from build123d import *

# Parameters (mm, degrees)
SKETCH1_W            = 812.8
SKETCH1_H            = 711.2
BOSS_EXTRUDE1_DEPTH  = 152.4
SKETCH2_W            = 609.6
SKETCH2_H            = 508
CUT_EXTRUDE1_DEPTH   = 152.4
SKETCH4_R            = 31.75
BOSS_EXTRUDE3_DEPTH  = 508
BOSS_EXTRUDE4_DEPTH  = 508
SKETCH7_R            = 31.75
BOSS_EXTRUDE5_DEPTH  = 508
BOSS_EXTRUDE6_DEPTH  = 508
BOSS_EXTRUDE7_DEPTH  = 508
SKETCH11_W           = 50.8
SKETCH11_H           = 508
BOSS_EXTRUDE8_DEPTH  = 76.2
CUT_EXTRUDE2_DEPTH   = 508
SKETCH14_W           = 609.6
SKETCH14_H           = 25.4
BOSS_EXTRUDE10_DEPTH = 50.8
SKETCH15_R           = 31.75
BOSS_EXTRUDE11_DEPTH = 508


with BuildPart() as part:
    # Sketch1 → Boss-Extrude1 (new body)
    with BuildSketch(Plane(origin=(0, 0, 0), x_dir=(1, 0, 0), z_dir=(0, 1, 0))):
        with Locations((406.4, -355.6)):
            Rectangle(SKETCH1_W, SKETCH1_H)
    extrude(amount=BOSS_EXTRUDE1_DEPTH)

    # Sketch2 → Cut-Extrude1 (cut)
    with BuildSketch(Plane(origin=(0, 152.4, 0), x_dir=(1, 0, 0), z_dir=(0, 1, 0))):
        with Locations((406.4, -355.6)):
            Rectangle(SKETCH2_W, SKETCH2_H)
    extrude(amount=-CUT_EXTRUDE1_DEPTH, mode=Mode.SUBTRACT)

    # Sketch4 → Boss-Extrude3 (add)
    with BuildSketch(Plane.XY.offset(101.6)):
        with Locations(Location((152.4, 25.4, 0), (0, 0, 233.130102354))):
            Circle(SKETCH4_R)
    extrude(amount=BOSS_EXTRUDE3_DEPTH)

    # Sketch6 → Boss-Extrude4 (add)
    with BuildSketch(Plane.XY.offset(101.6)):
        with BuildLine():
            Line((373.396614636, 28.575), (482.6, 152.4))
            Line((482.6, 152.4), (482.6, 0))
            Line((482.6, 0), (386.295833398, 0))
            ThreePointArc((386.295833398, 0), (382.921614636, 15.675781238), (373.396614636, 28.575))
        make_face()
    extrude(amount=BOSS_EXTRUDE4_DEPTH)

    # Sketch7 → Boss-Extrude5 (add)
    with BuildSketch(Plane.XY.offset(101.6)):
        with Locations(Location((348.195833398, 0, 0), (0, 0, 180))):
            Circle(SKETCH7_R)
    extrude(amount=BOSS_EXTRUDE5_DEPTH)

    # Sketch8 → Boss-Extrude6 (add)
    with BuildSketch(Plane.XY.offset(101.6)):
        Polygon((373.396614636, 28.575), (363.871614636, 36.975260413), (473.075, 160.800260413), (482.6, 152.4), align=None)
    extrude(amount=BOSS_EXTRUDE6_DEPTH)

    # Sketch9 → Boss-Extrude7 (add)
    with BuildSketch(Plane.XY.offset(609.6)):
        Polygon((482.6, 152.4), (641.222949159, 635), (631.697949159, 643.400260413), (473.075, 160.800260413), align=None)
    extrude(amount=-BOSS_EXTRUDE7_DEPTH)

    # Sketch11 → Boss-Extrude8 (add)
    with BuildSketch(Plane(origin=(379.25081554, -124.653714944, 0), x_dir=(0, 0, 1), z_dir=(-0.95, 0.3122498999199199, 0))):
        with Locations((584.2, 554.477868797)):
            Rectangle(SKETCH11_W, SKETCH11_H)
        with Locations((127, 554.477868797)):
            Rectangle(SKETCH11_W, SKETCH11_H)
    extrude(amount=BOSS_EXTRUDE8_DEPTH)

    # Sketch12 → Cut-Extrude2 (cut)
    with BuildSketch(Plane(origin=(0, 0, 101.6), x_dir=(-1, 0, 0), z_dir=(0, 0, -1))):
        Polygon((-579.47237543, 647.197555329), (-429.198002543, 189.997555329), (-453.328002543, 182.066407871), (-603.60237543, 639.266407871), align=None)
    extrude(amount=-CUT_EXTRUDE2_DEPTH, mode=Mode.SUBTRACT)

    # Sketch14 → Boss-Extrude10 (add)
    with BuildSketch(Plane(origin=(0, 152.4, 0), x_dir=(1, 0, 0), z_dir=(0, 1, 0))):
        with Locations((406.4, -88.9)):
            Rectangle(SKETCH14_W, SKETCH14_H)
        with Locations((406.4, -622.3)):
            Rectangle(SKETCH14_W, SKETCH14_H)
    extrude(amount=BOSS_EXTRUDE10_DEPTH)

    # Sketch15 → Boss-Extrude11 (add)
    with BuildSketch(Plane(origin=(0, 0, 609.6), x_dir=(-1, 0, 0), z_dir=(0, 0, -1))):
        with Locations(Location((-342.9, 127, 0), (0, 0, 180))):
            Circle(SKETCH15_R)
    extrude(amount=BOSS_EXTRUDE11_DEPTH)


solid = part.part
Source: CAD feature listing. Evaluate the final solid. Frame: model axes, mm. A direction names the side the tool comes from. Give positions to 0.01 mm unless a question says otherwise; leave off trailing zeros. Loops run counter-clockwise (first coordinate to the right, second up) from the corner with the lowest first, then second, coordinate; pieces in that order, holes last. Notation, with made-up numbers: (75.25, 57.25) -> (87.25, 57.25) arc R25 ccw to (87.25, 71.25) -> close; hole circle Ø4 at (8, -18). An arc over 180 degrees is marked (long way). Use a Markdown table: item, result. Add a question column.
1) First-contact query: pin 1 (3 mm diameter, centred on y = 247, z = 578.5, fed in from -X); pin 2 (2 mm diameter, centred on y = 262.5, z = 561, fed in from +X); pin 3 (1 mm diameter, centred on y = 558.5, z = 579, fed in from -X). Flat tips, straight axial feed; report the tip coordinate or a pass-through.
2) Line query: line 1 along X through (y, z) = (80, 330); line 2 along X through (y, z) = (134, 360); line 3 along Y through (x, z) = (715.5, 325.5). Output: solid intervals per line, ascending. Write a range as [from, to].
3) Section query D-D, the plane y = 127. Return the cut outline in (x, z).
4) Reachability of faces 5 (the face through (711.2, 77, 359)), 6 (the face through (541, 419, 101.6)), 7 (the face through (445, 195, 101.6)), 8 (the face through (101.6, 177, 89)), 9 (the face through (711.2, 177, 622)) from +Z, -Z, +X, -X, +Y, -Y: full face, straight path, thin tool, end or side. Return the list, or none.
5) Pull-direction query (X, two-part tool) for faces 1 (the face through (243, 103, 609.6)), 2 (the face through (505.387, 421.798, 126.644)), 3 (the face through (0, 75, 361)), 4 (the face through (401, 75, 0)); classes: +X half, -X half, draft (parallel to the pull), parting line (faces both ways), or undercut.
6) Section query C-C, the plane y = 399.5. Return the cut outline in (x, z).
7) Section query A-A, the plane x = 689. Return the cut outline in (y, z), then the cut area to 3 significant figures.
8) Section query B-B, the plane z = 331.5. Return the cut outline in (x, y) (3 decimals).
Numbers:
| question | item | result |
|---|---|---|
| 1 | pin 1 | stops at x = 420.7 |
| 1 | pin 2 | stops at x = 519.12 |
| 1 | pin 3 | stops at x = 523.42 |
| 2 | line 1 | x = [0, 101.6], [401.82, 482.6], [711.2, 812.8] |
| 2 | line 2 | x = [0, 101.6], [311.93, 373.87], [449.44, 482.6], [711.2, 812.8] |
| 2 | line 3 | y = [0, 152.4] |
| 3 | outline | (0, 0) -> (812.8, 0) -> (812.8, 711.2) -> (0, 711.2) -> close; hole (101.6, 101.6) -> (311.15, 101.6) -> (311.15, 609.6) -> (101.6, 609.6) -> close; hole (374.65, 101.6) -> (443.27, 101.6) -> (443.27, 609.6) -> (374.65, 609.6) -> close; hole (482.6, 101.6) -> (711.2, 101.6) -> (711.2, 609.6) -> (482.6, 609.6) -> close |
| 4 | face 5 | +Y, -Y |
| 4 | face 6 | -Z, +X, -X, +Y |
| 4 | face 7 | none |
| 4 | face 8 | +Z, -Z, -X, +Y |
| 4 | face 9 | +Z, -Z, +X, +Y |
| 5 | face 1 | undercut |
| 5 | face 2 | undercut |
| 5 | face 3 | -X half |
| 5 | face 4 | draft |
| 6 | outline | (471.32, 101.6) -> (498.06, 101.6) -> (498.06, 152.4) -> (471.32, 152.4) -> close; (471.32, 558.8) -> (498.06, 558.8) -> (498.06, 609.6) -> (471.32, 609.6) -> close; (524.79, 101.6) -> (563.82, 101.6) -> (563.82, 609.6) -> (524.79, 609.6) -> (524.79, 558.8) -> (551.53, 558.8) -> (551.53, 152.4) -> (524.79, 152.4) -> close |
| 7 | outline | (0, 0) -> (152.4, 0) -> (152.4, 76.2) -> (203.2, 76.2) -> (203.2, 101.6) -> (0, 101.6) -> close; (0, 609.6) -> (203.2, 609.6) -> (203.2, 635) -> (152.4, 635) -> (152.4, 711.2) -> (0, 711.2) -> close |
| 7 | area | 33,500 mm2 |
| 8 | outline | (0, 0) -> (101.6, 0) -> (101.6, 152.4) -> (0, 152.4) -> close; circle Ø63.5 at (152.4, 25.4); circle Ø63.5 at (342.9, 127); circle Ø63.5 at (348.196, 0); (363.872, 36.975) -> (373.397, 28.575) arc R38.1 cw to (386.296, 0) -> (482.6, 0) -> (482.6, 152.4) -> (641.223, 635) -> (631.698, 643.4) -> (473.075, 160.8) -> close; (711.2, 0) -> (812.8, 0) -> (812.8, 152.4) -> (711.2, 152.4) -> close |
